Input: part model. Units: mm. Frame: model coordinates. A direction names the side the tool comes from. Round coordinates to 2 decimals unless told otherwise and drop trailing zeros. Loops run counter-clockwise (first coordinate to the right, second up) from the corner with the lowest first, then second, coordinate; pieces in that order, holes last. Notation, with made-up numbers: M 42,35.5 L 82,35.5 A13 cw 82,43.5 Z; hole C 60.25,10.25 d9. An arc over 180 degrees is marked long. Put each result on its own line as item: value. Start each with the question number.
1) Line query: probe 1 along X at (y, z) = (45.5, 15.5); probe 2 along X at (y, z) = (33.5, 26). Output: solid intervals per line, ascending.
2) Section C-C on x = 37.5. Output: boundary loops of the cut face in (y, z).
3) Draft query along Z for faces 1 (the face through (48, -1, 30)), 2 (the face through (-48, 0, 8.115)), 3 (the face through (-1, 1, 4)). Return one class per face: +Z half, -Z half, draft (parallel to the pull), parting line (faces both ways), or undercut.
4) Section B-B on y = -1.5. Output: boundary loops of the cut face in (x, z).
5) Pin query (flat end, axial travel): pin 1 (6 mm diameter, centred on x = 6.5, z = 31, fed in from +Y); pin 2 (0.5 mm diameter, centred on x = 2, z = 3.5, fed in from -Y); pin 3 (5 mm diameter, centred on y = -12.5, z = 30, fed in from +X). Return the tip coordinate at first contact, or that it passes through.
6) Section A-A on z = 32.5. Output: boundary loops of the cut face in (x, y), plus the area to 3 significant figures.
7) Reachability of faces 4 (the face through (-48, 0, 3.115)), 5 (the face through (-1, 46, 19)), 6 (the face through (-48, -1, 30)) from +Z, -Z, +X, -X, +Y, -Y: full face, straight path, thin tool, end or side. Return the list, or none.
from build123d import *

# Parameters (mm, degrees)
F0_W     = 100
F0_H     = 100
F1_DEPTH = 35
F2_T     = -4
F3_W     = 96
F3_H     = 96
F4_DEPTH = 10
F5_W     = 30
F5_H     = 5
F6_DEPTH = 5
F8_DEPTH = 5


with BuildPart() as f1:
    # F0 (on Top) → F1 (new body)
    with BuildSketch(Plane.XY):
        Rectangle(F0_W, F0_H)
    extrude(amount=F1_DEPTH)

    # F2
    f2_openings = [f1.faces().sort_by_distance(p)[0] for p in [
        (0, 0, 35),
    ]]
    offset(amount=F2_T, openings=f2_openings)

    # F3 (on face) → F4 (cut)
    with BuildSketch(Plane.XY.offset(35)):
        Polygon((-48, 50), (-50, 50), (-50, 48), (-50, -48), (-50, -50), (-48, -50), (48, -50), (50, -50), (50, -48), (50, 48), (50, 50), (48, 50), align=None)
        Rectangle(F3_W, F3_H, mode=Mode.SUBTRACT)
    extrude(amount=-F4_DEPTH, mode=Mode.SUBTRACT)

    # F5 (on face) → F6 (cut)
    with BuildSketch(Plane(origin=(-50, 0, 0), x_dir=(0, -1, 0), z_dir=(-1, 0, 0))):
        with Locations((0, 5.614583)):
            Rectangle(F5_W, F5_H)
    extrude(amount=-F6_DEPTH, mode=Mode.SUBTRACT)

    # F7 (on face) → F8 (cut)
    with BuildSketch(Plane.XZ.offset(50)):
        with BuildLine():
            add(Edge.make_bspline(
                [(-10, 9.723425), (-10, -3.266956), (5, 3.228234), (20, 9.723425), (5, 16.218615), (-10, 22.713806), (-10, 9.723425)],
                knots=[0, 0, 0, 2.094395, 2.094395, 4.18879, 4.18879, 6.283185, 6.283185, 6.283185], degree=2, weights=[1, 0.5, 1, 0.5, 1, 0.5, 1]))
        make_face()
    extrude(amount=-F8_DEPTH, mode=Mode.SUBTRACT)


solid = f1.part
Geometry results:
1. probe 1: x = -50 to -46, 46 to 50
1. probe 2: x = -48 to -46, 46 to 48
2. outline: M -50,0 L 50,0 L 50,25 L 48,25 L 48,35 L 46,35 L 46,4 L -46,4 L -46,35 L -48,35 L -48,25 L -50,25 Z
3. face 1: draft
3. face 2: undercut
3. face 3: +Z half
4. outline: M -50,0 L 50,0 L 50,25 L 48,25 L 48,35 L 46,35 L 46,4 L -45,4 L -45,3.11 L -50,3.11 Z; M -50,8.11 L -46,8.11 L -46,35 L -48,35 L -48,25 L -50,25 Z
5. pin 1: stops at y = 48
5. pin 2: stops at y = -45
5. pin 3: stops at x = 48
6. outline: M -48,-48 L 48,-48 L 48,48 L -48,48 Z; hole M -46,-46 L 46,-46 L 46,46 L -46,46 Z
6. area: 752 mm²
7. face 4: -X
7. face 5: +Z
7. face 6: +Z, -X, +Y, -Y
